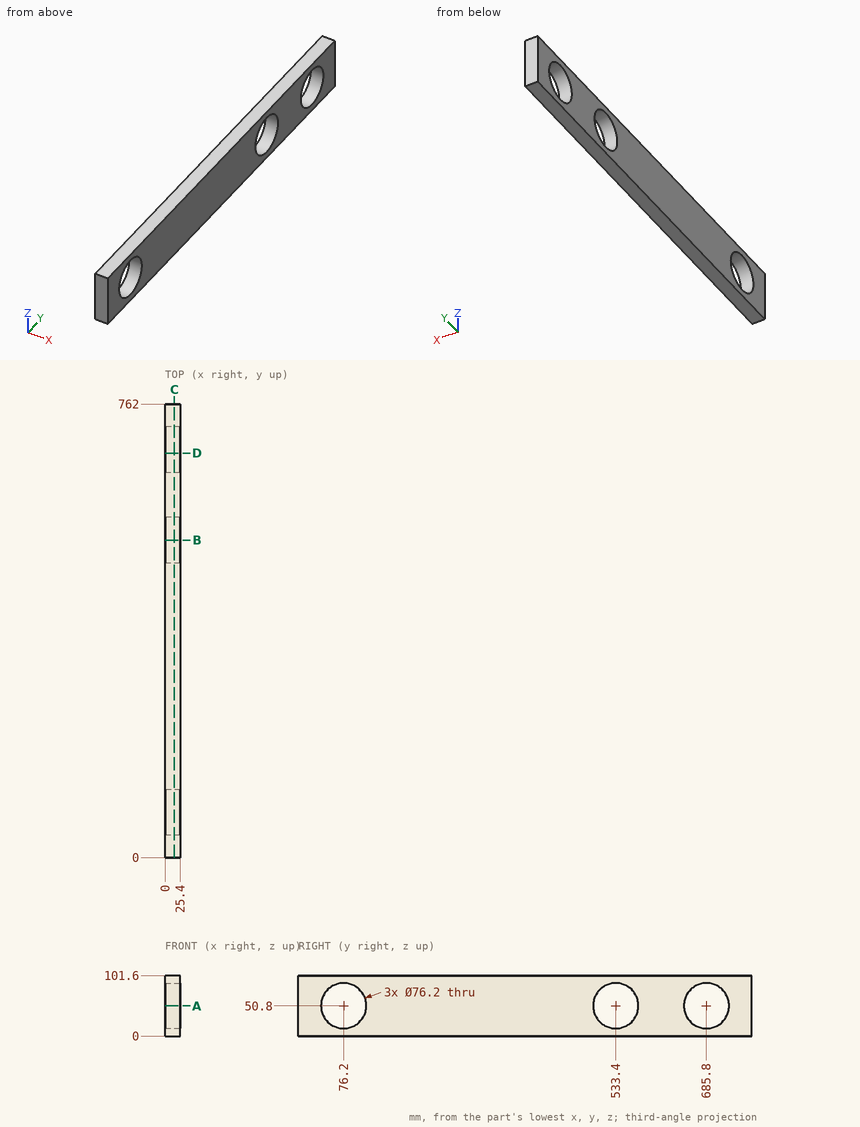
Print and shaded views of the part. All mm, measured from the part's lowest x, y and z. Coordinates: 2 decimals unless noted, no trailing zeros. Order: outer loops, then holes, each group sorted by start corner. A loop starts at its lowest first (then second) coordinate and runs counter-clockwise, first axis right, second up. Notation, with made-up numbers: (-16.5, 66) - (15.5, 66) arc R21 ccw to (15.5, 77) - close; hole circle Ø8 at (52, 53.5). An arc over 180 degrees is marked (long way). Put each result on its own line as item: value.
1. Saw through at A-A (z = 50.8). Write the cut outline in (x, y).
Answer sheet:
outline: (0, 0) - (25.4, 0) - (25.4, 38.1) - (0, 38.1) - close; (0, 114.3) - (25.4, 114.3) - (25.4, 495.3) - (0, 495.3) - close; (0, 571.5) - (25.4, 571.5) - (25.4, 647.7) - (0, 647.7) - close; (0, 723.9) - (25.4, 723.9) - (25.4, 762) - (0, 762) - close
2. Probe line 1 along Y through (x, z) = (21.5, 53); line 2 along Z through (x, y) = (14.25, 76.2); line 3 along Y through (x, z) = (14.5, 60.5). List the from-to ranges inside material, lowest first. Write a range as [from, to].
Answer sheet:
line 1: y = [0, 38.16], [114.24, 495.36], [571.44, 647.76], [723.84, 762]
line 2: z = [0, 12.7], [88.9, 101.6]
line 3: y = [0, 39.36], [113.04, 496.56], [570.24, 648.96], [722.64, 762]
3. Saw through at B-B (y = 533.4). Write the cut outline in (x, z).
Answer sheet:
outline: (0, 0) - (25.4, 0) - (25.4, 12.7) - (0, 12.7) - close; (0, 88.9) - (25.4, 88.9) - (25.4, 101.6) - (0, 101.6) - close
4. Saw through at C-C (x = 15.5). Write the cut outline in (y, z).
Answer sheet:
outline: (0, 0) - (762, 0) - (762, 101.6) - (0, 101.6) - close; hole circle Ø76.2 at (76.2, 50.8); hole circle Ø76.2 at (533.4, 50.8); hole circle Ø76.2 at (685.8, 50.8)
5. Saw through at D-D (y = 679.5). Write the cut outline in (x, z), and give its area (3 significant figures).
Answer sheet:
outline: (0, 0) - (25.4, 0) - (25.4, 13.22) - (0, 13.22) - close; (0, 88.38) - (25.4, 88.38) - (25.4, 101.6) - (0, 101.6) - close
area: 672 mm^2
